```python
from build123d import *

# Parameters (mm, degrees)
SKETCH1_W               = 220
SKETCH1_H               = 240
SKETCH1_R               = 1.5
SKETCH1_W_2             = 19
SKETCH1_H_2             = 35
BOSS_EXTRUDE1_DEPTH     = 10
CUT_EXTRUDE1_DEPTH      = 164.095064303
CUT_EXTRUDE1_DEPTH_BACK = 3
SKETCH2_W               = 147
SKETCH2_H               = 55
SKETCH3_W               = 34
SKETCH3_H               = 55
BOSS_EXTRUDE2_DEPTH     = 3
SKETCH6_W               = 2.5
SKETCH6_H               = 35
CUT_EXTRUDE3_DEPTH      = 10
SKETCH7_W               = 2
SKETCH7_H               = 35
CUT_EXTRUDE4_DEPTH      = 10


with BuildPart() as part:
    # Sketch1 → Boss-Extrude1 (new body)
    with BuildSketch(Plane.XY):
        Rectangle(SKETCH1_W, SKETCH1_H)
        with Locations((18.8, -40)):
            Circle(SKETCH1_R, mode=Mode.SUBTRACT)
        with Locations((45.8, -40)):
            Circle(SKETCH1_R, mode=Mode.SUBTRACT)
        with Locations((45.8, -105)):
            Circle(SKETCH1_R, mode=Mode.SUBTRACT)
        with Locations((18.8, -105)):
            Circle(SKETCH1_R, mode=Mode.SUBTRACT)
        with Locations((-45.8, 105)):
            Circle(SKETCH1_R, mode=Mode.SUBTRACT)
        with Locations((-18.8, 105)):
            Circle(SKETCH1_R, mode=Mode.SUBTRACT)
        with Locations((-18.8, 40)):
            Circle(SKETCH1_R, mode=Mode.SUBTRACT)
        with Locations((-45.8, 40)):
            Circle(SKETCH1_R, mode=Mode.SUBTRACT)
        with Locations((-80, 0)):
            Circle(SKETCH1_R, mode=Mode.SUBTRACT)
        with Locations((80, 0)):
            Circle(SKETCH1_R, mode=Mode.SUBTRACT)
        with Locations((90, 86.169859373)):
            Circle(SKETCH1_R, mode=Mode.SUBTRACT)
        with Locations((90, 65.169859373)):
            Circle(SKETCH1_R, mode=Mode.SUBTRACT)
        with Locations((107, 65.169859373)):
            Circle(SKETCH1_R, mode=Mode.SUBTRACT)
        with Locations((107, 86.169859373)):
            Circle(SKETCH1_R, mode=Mode.SUBTRACT)
        with Locations((90, -10.5)):
            Circle(SKETCH1_R, mode=Mode.SUBTRACT)
        with Locations((90, 10.5)):
            Circle(SKETCH1_R, mode=Mode.SUBTRACT)
        with Locations((107, 10.5)):
            Circle(SKETCH1_R, mode=Mode.SUBTRACT)
        with Locations((107, -10.5)):
            Circle(SKETCH1_R, mode=Mode.SUBTRACT)
        with Locations((90, -86.169859373)):
            Circle(SKETCH1_R, mode=Mode.SUBTRACT)
        with Locations((90, -65.169859373)):
            Circle(SKETCH1_R, mode=Mode.SUBTRACT)
        with Locations((107, -65.169859373)):
            Circle(SKETCH1_R, mode=Mode.SUBTRACT)
        with Locations((107, -86.169859373)):
            Circle(SKETCH1_R, mode=Mode.SUBTRACT)
        with Locations((-107, -65.169859373)):
            Circle(SKETCH1_R, mode=Mode.SUBTRACT)
        with Locations((-107, -86.169859373)):
            Circle(SKETCH1_R, mode=Mode.SUBTRACT)
        with Locations((-90, -86.169859373)):
            Circle(SKETCH1_R, mode=Mode.SUBTRACT)
        with Locations((-90, -65.169859373)):
            Circle(SKETCH1_R, mode=Mode.SUBTRACT)
        with Locations((-107, -10.5)):
            Circle(SKETCH1_R, mode=Mode.SUBTRACT)
        with Locations((-107, 10.5)):
            Circle(SKETCH1_R, mode=Mode.SUBTRACT)
        with Locations((-90, 10.5)):
            Circle(SKETCH1_R, mode=Mode.SUBTRACT)
        with Locations((-90, -10.5)):
            Circle(SKETCH1_R, mode=Mode.SUBTRACT)
        with Locations((-107, 86.169859373)):
            Circle(SKETCH1_R, mode=Mode.SUBTRACT)
        with Locations((-107, 65.169859373)):
            Circle(SKETCH1_R, mode=Mode.SUBTRACT)
        with Locations((-90, 65.169859373)):
            Circle(SKETCH1_R, mode=Mode.SUBTRACT)
        with Locations((-90, 86.169859373)):
            Circle(SKETCH1_R, mode=Mode.SUBTRACT)
        with Locations((-59, 0)):
            Rectangle(SKETCH1_W_2, SKETCH1_H_2, mode=Mode.SUBTRACT)
        with Locations((59, 0)):
            Rectangle(SKETCH1_W_2, SKETCH1_H_2, mode=Mode.SUBTRACT)
        Rectangle(SKETCH1_W_2, SKETCH1_H_2, mode=Mode.SUBTRACT)
    extrude(amount=BOSS_EXTRUDE1_DEPTH)

    # Sketch2 → Cut-Extrude1 (cut, two sides: drawn at the far end of the back side and taken through both)
    with BuildSketch(Plane.XY.offset(10).offset(-CUT_EXTRUDE1_DEPTH_BACK)):
        Rectangle(SKETCH2_W, SKETCH2_H)
    extrude(amount=CUT_EXTRUDE1_DEPTH + CUT_EXTRUDE1_DEPTH_BACK, mode=Mode.SUBTRACT)

    # Sketch3 → Boss-Extrude2 (add)
    with BuildSketch(Plane.XY.offset(7)):
        with Locations((29.5, 0)):
            Rectangle(SKETCH3_W, SKETCH3_H)
        with Locations((-29.5, 0)):
            Rectangle(SKETCH3_W, SKETCH3_H)
    extrude(amount=BOSS_EXTRUDE2_DEPTH)

    # Sketch6 → Cut-Extrude3 (cut)
    with BuildSketch(Plane.XY.offset(7)):
        with Locations((-69.75, 0)):
            Rectangle(SKETCH6_W, SKETCH6_H)
        with Locations((69.75, 0)):
            Rectangle(SKETCH6_W, SKETCH6_H)
    extrude(amount=-CUT_EXTRUDE3_DEPTH, mode=Mode.SUBTRACT)

    # Sketch7 → Cut-Extrude4 (cut)
    with BuildSketch(Plane.XY.offset(7)):
        with Locations((10.5, 0)):
            Rectangle(SKETCH7_W, SKETCH7_H)
        with Locations((-10.5, 0)):
            Rectangle(SKETCH7_W, SKETCH7_H)
    extrude(amount=-CUT_EXTRUDE4_DEPTH, mode=Mode.SUBTRACT)


solid = part.part
```
For this review, take the finished solid that the model builds, in its own axes (mm). A direction names the side the tool comes from. Give positions to 0.01 mm unless a question says otherwise; leave off trailing zeros. Write each loop counter-clockwise with the first axis right and the second up, starting at its lowest first coordinate (ties: lowest second). Pieces come first, ordered by that corner, then holes. Notation, with made-up numbers: M 44.5,45.5 L 53.5,45.5 A15 cw 53.5,68.5 Z; hole C 45.5,2 d1. An arc over 180 degrees is marked long. Answer as a JSON object with one key per item and string values. Group by question number.
Item 1: Consider section A-A on x = -7. Write out the cut boundary in (y, z).
Item 2: For probe 1 along X at (y, z) = (-105, 8); probe 2 along Y at (x, z) = (-69.5, 0.5); probe 3 along X at (y, z) = (-2, 3), list the stretches that pass through material, from the lowest coordinate up. Write a range as [from, to].
Item 3: For pin 1 Ø8 at (x, y) = (57.5, 17.5) entering from +Z; pin 2 Ø1.8 at (x, y) = (-90, -10.5) entering from +Z, all flat-tipped, find the tip position at first contact; note any pin that passes through.
Item 4: Tool access review of faces 1 (the flat face through (23, 2, 0)), 2 (the flat face through (49.5, 0, 3)), 3 (the flat face through (72, 0, 7)): name each direction out of +Z, -Z, +X, -X, +Y, -Y from which nothing blocks a thin tool from reaching the whole face with its end or side.
Item 5: Draft analysis for pull direction X (two halves, no side actions). For faces 4 (the flat face through (0, 19, 7)), 5 (the flat face through (110, -2, 5)), 6 (the flat face through (-2, -120, 5)), 7 (the flat face through (-110, -2, 5)), state which applies: +X half, -X half, draft (parallel to the pull), parting line (faces both ways), or undercut.
Item 6: Consider section B-B on z = 2.25. Count the separate pieces of the cut face and the enclosed holes in it, plus the area to 3 significant figures.
Check result:
{
 "1": {"outline": "M -120,0 L -17.5,0 L -17.5,7 L -27.5,7 L -27.5,10 L -120,10 Z; M 17.5,0 L 120,0 L 120,10 L 27.5,10 L 27.5,7 L 17.5,7 Z"},
 "2": {"probe 1": "x = [-110, 17.3], [20.3, 44.3], [47.3, 110]", "probe 2": "y = [-120, -17.5], [17.5, 120]", "probe 3": "x = [-110, -71], [-49.5, -11.5], [11.5, 49.5], [71, 110]"},
 "3": {"pin 1": "stops at z = 7", "pin 2": "passes through"},
 "4": {"face 1": "-Z, +X, -X, +Y, -Y", "face 2": "+Z, -Z", "face 3": "+Z"},
 "5": {"face 4": "undercut", "face 5": "+X half", "face 6": "draft", "face 7": "-X half"},
 "6": {"separate pieces": "1", "enclosed holes": "37", "area": "50,200 mm^2"}
}
